Can you work these out from the model? Positions are in its coordinate system, mm. A direction names the side the tool comes from. Give positions to 0.01 mm unless a question says otherwise; leave off trailing zeros. Order: outer loops, then holes, each group sorted by start corner. A loop starts at its lowest first (then second) coordinate and runs counter-clockwise, first axis right, second up. Notation, with made-up numbers: (87, 69) - (144, 69) arc R6 ccw to (144, 79) - close; hole circle Ø5 at (40, -10). An arc over 180 degrees is marked (long way). Use one line per item in the form item = value. Start each with the question number.
1) Please list where these lines run through material, in increasing order: probe 1 along Y at (x, z) = (-7, -5); probe 2 along Z at (x, y) = (-59, -27) (3 decimals); probe 3 along X at (y, z) = (-35, 12) (3 decimals).
2) Suppose I cut it at B-B, the plane y = 56. Write out the boundary of the cut face in (x, z) (3 decimals).
3) For pin 1 (4 mm diameter, centred on x = 16.5, z = 12, fed in from +Y); pin 2 (21 mm diameter, centred on y = -45.5, z = -14.5, fed in from -X) (3 decimals); pin 3 (3.5 mm diameter, centred on x = -41, z = -1, fed in from -Y), each with a flat end and sliding along its axis, tell me the tip position at first contact or that it passes through.
4) We'd pull the mould along Y, two halves only. Please class faces 1 (the flat face through (0, 31.75, -9)), 2 (the flat face through (0, -76.2, 8)), 3 (the flat face through (-16, 48, 12.7)), 4 (the flat face through (0, 76.2, -8)): released by +Y, released by -Y, zero draft, split by the parting line, or undercut.
5) Suppose I cut it at C-C, the plane y = -6. Write out the boundary of the cut face in (x, z) (3 decimals), and give its area (3 significant figures).
6) Which directions (+Z, -Z, +X, -X, +Y, -Y) give clear straight access to the entire face, cutting with the end or side of a thin tool? Please do faces 5 (the flat face through (0, 47, 6)), 6 (the flat face through (0, 70, -12.7)), 7 (the flat face through (-16, 63.5, 6)), 8 (the flat face through (-28.575, -39, -13)), 9 (the flat face through (-28.575, -39, 8)).
7) Suppose I cut it at D-D, the plane x = -23. Write out the boundary of the cut face in (y, z) (3 decimals), and give its area (3 significant figures).
```python
from build123d import *

# Parameters (mm, degrees)
F0_R      = 82.55
F2_DEPTH  = 3.175
F1_W      = 57.15
F1_H      = 76.2
F3_DEPTH  = 15.875
F4_DEPTH  = 22.225
F5_DEPTH  = 12.7
F6_DEPTH  = 12.7
F7_DEPTH  = 15.875
F9_DEPTH  = 12.7
F10_DEPTH = 25.4


with BuildPart() as f2:
    # F0 (on Top) → F2 (new body)
    with BuildSketch(Plane.XY):
        Circle(F0_R)
    extrude(amount=-F2_DEPTH)

    # F1 (on Top) → F3 (join)
    with BuildSketch(Plane.XY):
        with Locations((0, -38.1)):
            Rectangle(F1_W, F1_H)
    extrude(amount=F3_DEPTH)

    # F1 (on Top) → F4 (join)
    with BuildSketch(Plane.XY):
        with Locations((0, -38.1)):
            Rectangle(F1_W, F1_H)
    extrude(amount=-F4_DEPTH)

    # F1 (on Top) → F5 (join)
    with BuildSketch(Plane.XY):
        Polygon((-31.75, 76.2), (-31.75, 63.5), (0, 63.5), (31.75, 63.5), (31.75, 76.2), align=None)
    extrude(amount=-F5_DEPTH)

    # F1 (on Top) → F6 (join)
    with BuildSketch(Plane.XY):
        Polygon((0, 63.5), (-31.75, 63.5), (-31.75, 31.75), (-26.9875, 31.75), (0, 31.75), align=None)
    extrude(amount=F6_DEPTH)

    # F1 (on Top) → F7 (join)
    with BuildSketch(Plane.XY):
        Polygon((26.9875, 31.75), (0, 31.75), (-26.9875, 31.75), (-26.9875, 6.35), (26.9875, 6.35), align=None)
    extrude(amount=F7_DEPTH)

    # F8 (on face) → F9 (join)
    with BuildSketch(Plane(origin=(0, 0, -3.175), x_dir=(1, 0, 0), z_dir=(0, 0, -1))):
        Polygon((-28.575, 0), (-31.75, 0), (-31.75, -31.75), (31.75, -31.75), (31.75, 0), (28.575, 0), align=None)
    extrude(amount=F9_DEPTH)

    # F8 (on face) → F10 (cut)
    with BuildSketch(Plane(origin=(0, 0, -3.175), x_dir=(1, 0, 0), z_dir=(0, 0, -1))):
        Polygon((31.75, 0), (31.75, -31.75), (44.45, -31.75), (44.45, 19.05), (31.75, 19.05), align=None)
        Polygon((-31.75, -31.75), (-31.75, 0), (-31.75, 19.05), (-44.45, 19.05), (-44.45, -63.5), (-31.75, -63.5), align=None)
    extrude(amount=-F10_DEPTH, mode=Mode.SUBTRACT)


solid = f2.part
```
Result sheet:
q1.probe_1 = -76.2 to 31.75, 63.5 to 76.2
q1.probe_2 = -3.175 to 0
q1.probe_3 = -28.575 to 28.575
q2.outline = (-60.651, -3.175) - (-44.45, -3.175) - (-44.45, 0) - (-60.651, 0) - close; (-31.75, -3.175) - (60.651, -3.175) - (60.651, 0) - (0, 0) - (0, 12.7) - (-31.75, 12.7) - close
q3.pin_1 = 31.75
q3.pin_2 = -28.575
q3.pin_3 = -72.62
q4.face_1 = undercut
q4.face_2 = released by -Y
q4.face_3 = zero draft
q4.face_4 = released by +Y
q5.outline = (-82.332, -3.175) - (-44.45, -3.175) - (-44.45, 0) - (-82.332, 0) - close; (-31.75, -3.175) - (-28.575, -3.175) - (-28.575, -22.225) - (28.575, -22.225) - (28.575, -3.175) - (31.75, -3.175) - (31.75, 0) - (28.575, 0) - (28.575, 15.875) - (-28.575, 15.875) - (-28.575, 0) - (-31.75, 0) - close; (44.45, -3.175) - (82.332, -3.175) - (82.332, 0) - (44.45, 0) - close
q5.area = 2,440 mm²
q6.face_5 = +Z, +X, +Y
q6.face_6 = -Z, +X, -X, +Y
q6.face_7 = +Z, +X, -X, +Y
q6.face_8 = -Z, -X, -Y
q6.face_9 = +Z, -X, -Y
q7.outline = (-79.281, -3.175) - (-76.2, -3.175) - (-76.2, -22.225) - (0, -22.225) - (0, -15.875) - (31.75, -15.875) - (31.75, -3.175) - (63.5, -3.175) - (63.5, -12.7) - (76.2, -12.7) - (76.2, -3.175) - (79.281, -3.175) - (79.281, 0) - (63.5, 0) - (63.5, 12.7) - (31.75, 12.7) - (31.75, 15.875) - (6.35, 15.875) - (6.35, 0) - (0, 0) - (0, 15.875) - (-76.2, 15.875) - (-76.2, 0) - (-79.281, 0) - close
q7.area = 4,500 mm²
